Geometry check sheet. Reference: the model listing, model coordinates, mm. Face numbers are marked on the shaded views. Give positions to 0.01 mm unless a question says otherwise; leave off trailing zeros. Write each loop counter-clockwise with the first axis right and the second up, starting at its lowest first coordinate (ties: lowest second). Pieces come first, ordered by that corner, then holes. Notation, with made-up numbers: (31, 34.5) - (57, 34.5) arc R29 cw to (57, 65.5) - close; hole circle Ø9 at (86, 34). An arc over 180 degrees is marked (long way). Use a Markdown table: item, result.
Solid Edge part; units mm, degrees
sketch "Sketch1" plane through (0, 0, 0) normal (0, 0, 1) x (1, 0, 0)
  line L0 (-35, -40) -> (35, -40)
  line L1 (35, -40) -> (35, 40)
  line L2 (35, 40) -> (-35, 40)
  line L3 (-35, 40) -> (-35, -40)
  dimension "D1" = 35
  dimension "D2" = 35
extrude "Protrusion1" add sketch "Sketch1" along normal blind 5
sketch "Sketch2" plane through (0, 0, 5) normal (0, 0, 1) x (1, 0, 0)
  circle A0 centre (-25, 34) radius 1.6
  dimension "D1" = 25
extrude "Cutout1" cut sketch "Sketch2" against normal through all
mirror "Mirror1" about plane through (0, 0, 0) normal (1, 0, 0) of "Cutout1"
mirror "Mirror2" about plane through (0, 0, 0) normal (0, -1, 0) of "Cutout1", "Mirror1"
sketch "Sketch3" plane through (0, 0, 5) normal (0, 0, 1) x (1, 0, 0)
  circle A0 centre (-13.5, 0) radius 1.5
extrude "Cutout2" cut sketch "Sketch3" against normal through all
mirror "Mirror3" about plane through (0, 0, 0) normal (1, 0, 0) of "Cutout2"
sketch "Sketch4" plane through (0, 0, 5) normal (0, 0, 1) x (1, 0, 0)
  line L0 (-33, 23) -> (-15, 23)
  line L1 (-15, 23) -> (-15, 25)
  line L2 (-15, 25) -> (-33, 25)
  line L3 (-33, 25) -> (-33, 23)
  dimension "D1" = 15
  dimension "D2" = 15
extrude "Extrusionsausprägung_2" add sketch "Sketch4" along normal blind 2
mirror "Mirror4" about plane through (0, 0, 0) normal (0, -1, 0) of "Extrusionsausprägung_2"
mirror "Mirror5" about plane through (0, 0, 0) normal (1, 0, 0) of "Mirror4", "Extrusionsausprägung_2"
fillet "Verrundung_1" radius 4 4 edges at (0, 40, 0) (35, 0, 0) (-35, 0, 0) (0, -40, 0)
fillet "Verrundung_2" radius 4 8 edges at (33.8284, 38.8284, 1.1716) (35, 40, 4.5) (33.8284, -38.8284, 1.1716) (35, -40, 4.5) (-33.8284, -38.8284, 1.1716) (-35, -40, 4.5) (-33.8284, 38.8284, 1.1716) (-35, 40, 4.5)
chamfer "Fase_1" distance 0.5 angle 60 2 edges at (15, 0, 5) (-15, 0, 5) measured on face at (-24.0333, -25.8667, 5)
chamfer "Fase_2" distance 0.5 angle 60 4 edges at (26.6, -34, 5) (-26.6, -34, 5) (-26.6, 34, 5) (26.6, 34, 5) measured on face at (-24.0333, -25.8667, 5)
properties material "Nylon, allgemein"
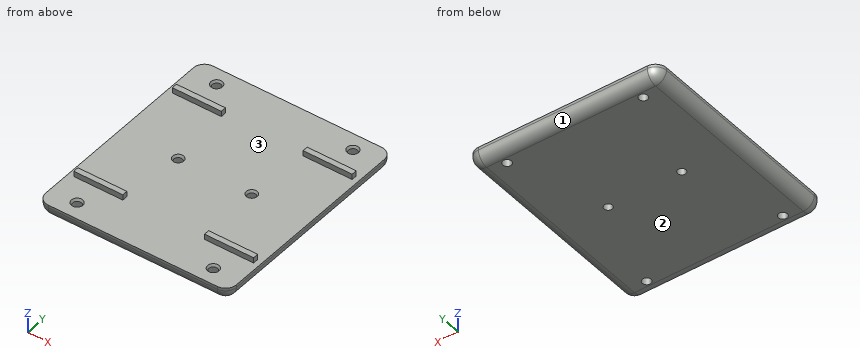
1) Section check B-B on x = 13.5. Record the boundary of the cut face in (y, z).
Working result:
| item | result |
|---|---|
| outline | (-40, 4) arc R4 ccw to (-36, 0) - (-1.5, 0) - (-1.5, 4.13) - (-2, 5) - (-40, 5) - close; (1.5, 0) - (36, 0) arc R4 ccw to (40, 4) - (40, 5) - (2, 5) - (1.5, 4.13) - close |
2) Section check C-C on x = 25. Record the boundary of the cut face in (y, z).
Working result:
| item | result |
|---|---|
| outline | (-40, 4) arc R4 ccw to (-36, 0) - (-35.6, 0) - (-35.6, 4.13) - (-36.1, 5) - (-40, 5) - close; (-32.4, 0) - (32.4, 0) - (32.4, 4.13) - (31.9, 5) - (25, 5) - (25, 7) - (23, 7) - (23, 5) - (-23, 5) - (-23, 7) - (-25, 7) - (-25, 5) - (-31.9, 5) - (-32.4, 4.13) - close; (35.6, 0) - (36, 0) arc R4 ccw to (40, 4) - (40, 5) - (36.1, 5) - (35.6, 4.13) - close |
3) Mould release check, pull along Y, two halves, no side actions. Record for the marked faces 1, 2 and 3: pulls with the +Y half, pulls with the -Y half, needs draft (parallel to the pull), parting line crosses it, or undercut.
Working result:
| item | result |
|---|---|
| face 1 | pulls with the +Y half |
| face 2 | needs draft |
| face 3 | undercut |
4) Depth check by flat-ended pin: P1, Ø1, axis at y = 24, z = 6, coming from the +X side; P2, Ø1, axis at y = -24, z = 6, coming from the -X side; P3, Ø1, axis at x = 27, z = 6, coming from the +Y side. Enter the tip coordinate at first touch or a pass-through.
Working result:
| item | result |
|---|---|
| P1 | stops at x = 33 |
| P2 | stops at x = -33 |
| P3 | stops at y = 25 |
5) Section check D-D on z = 1. Record the boundary of the cut face in (x, y).
Working result:
| item | result |
|---|---|
| outline | (-33.65, -36) arc R2.65 ccw to (-31, -38.65) - (31, -38.65) arc R2.65 ccw to (33.65, -36) - (33.65, 36) arc R2.65 ccw to (31, 38.65) - (-31, 38.65) arc R2.65 ccw to (-33.65, 36) - close; hole circle Ø3.2 at (-25, -34); hole circle Ø3.2 at (-25, 34); hole circle Ø3 at (-13.5, 0); hole circle Ø3 at (13.5, 0); hole circle Ø3.2 at (25, -34); hole circle Ø3.2 at (25, 34) |
6) Section check A-A on y = 34. Record the boundary of the cut face in (x, z).
Working result:
| item | result |
|---|---|
| outline | (-35, 4) arc R4 ccw to (-31, 0) - (-26.6, 0) - (-26.6, 4.13) - (-27.1, 5) - (-35, 5) - close; (-23.4, 0) - (23.4, 0) - (23.4, 4.13) - (22.9, 5) - (-22.9, 5) - (-23.4, 4.13) - close; (26.6, 0) - (31, 0) arc R4 ccw to (35, 4) - (35, 5) - (27.1, 5) - (26.6, 4.13) - close |
7) Material ranges on L1, parallel to Y at x = -18, z = 6; L2, parallel to Y at x = 25, z = 1; L3, parallel to X at y = -34, z = 1.9, recorded low to high. Write a range as from..to.
Working result:
| item | result |
|---|---|
| L1 | y = -25..-23, 23..25 |
| L2 | y = -38.65..-35.6, -32.4..32.4, 35.6..38.65 |
| L3 | x = -34.4..-26.6, -23.4..23.4, 26.6..34.4 |
